Can you work these out from the model? Positions are in its coordinate system, mm. A direction names the side the tool comes from. Give positions to 0.01 mm unless a question says otherwise; leave off trailing zeros. Write each loop counter-clockwise with the first axis right and the second up, starting at its lowest first coordinate (ties: lowest second). Pieces come first, ordered by that corner, then holes.
1. Suppose I cut it at B-B (z = 23.5). Please give me the cut outline in (x, y), and give its area (3 significant figures).
2. On a 3-axis mill with a long thin cutter (end or side, diameter ignored), from which of +Z, -Z, +X, -X, +Y, -Y can I reach the whole of each face in a straight line? I mean faces 1 (the cylindrical face through (8.396, -2.644, 36.442)), 2 (the flat face through (12, 5, 8.96)), 3 (the flat face through (0, 0, 0)). Say none if no direction works.
3. If I drill on probe 1 along Y at (x, z) = (7.5, 38.5); probe 2 along X at (y, z) = (1, 36.5); probe 3 along Z at (x, y) = (-12.5, 3.5), over which ranges is the centre line in solid material (lowest first)?
4. I'm going to push flat-ended pins straight in: pin 1 (10 mm diameter, centred on x = -6.5, y = -24.5, fed in from +Z); pin 2 (4 mm diameter, centred on x = -4.5, y = -15.5, fed in from -Z); pin 3 (3 mm diameter, centred on x = -10.5, z = 15, fed in from +Y). Where does each tip first touch, or does it pass through?
5. Suppose I cut it at A-A (z = 45). Please give me the cut outline in (x, y), and give its area (3 significant figures).
```python
from build123d import *


with BuildPart() as f1:
    # F0 (on Front) → F1 (revolve)
    with BuildSketch(Plane.XZ):
        with BuildLine():
            Line((0, 54.230746), (0, 0))
            Line((0, 0), (4.58643, 0))
            ThreePointArc((4.58643, 0), (8.098913, 1.059918), (10.438815, 3.885839))
            Line((10.438815, 3.885839), (12.575245, 8.959862))
            Line((12.575245, 8.959862), (25.716878, 8.959862))
            ThreePointArc((25.716878, 8.959862), (30.207006, 10.819734), (32.066878, 15.309862))
            Line((32.066878, 15.309862), (32.066878, 16.50501))
            Line((32.066878, 16.50501), (8.802673, 24.678919))
            Line((8.802673, 24.678919), (8.802673, 47.880746))
            ThreePointArc((8.802673, 47.880746), (6.942801, 52.370874), (2.452673, 54.230746))
            Line((2.452673, 54.230746), (0, 54.230746))
        make_face()
    revolve(axis=Axis((0, 0, 27.115373), (0, 0, -1)))


solid = f1.part
```
Checks:
1. outline: circle Ø24.32 at (0, 0)
1. area: 464 mm2
2. face 1: +Z
2. face 2: -Z
2. face 3: -Z, +X, -X, +Y, -Y
3. probe 1: y = -4.61 to 4.61
3. probe 2: x = -8.75 to 8.75
3. probe 3: z = 8.96 to 23.21
4. pin 1: stops at z = 20.62
4. pin 2: stops at z = 8.96
4. pin 3: stops at y = 30.77
5. outline: circle Ø17.61 at (0, 0)
5. area: 243 mm2
